Input: part model. Units: mm. Frame: model coordinates. Face numbers are marked on the shaded views. A direction names the side the tool comes from. Coordinates: 2 decimals unless noted, no trailing zeros. Write each loop counter-clockwise with the first axis right and the second up, starting at its lowest first coordinate (ties: lowest second). Pieces come first, ordered by that corner, then holes. Notation, with made-up numbers: (-38, 69) - (5, 69) arc R23 cw to (5, 102) - close; hole circle Ø9 at (-4, -32). An arc over 180 degrees is marked (long way). Put each result on its own line as item: value. Start each with the question number.
1. Cut plane A-A, the plane x = 7.5. Return loops of the section in (y, z), and give its area (3 significant figures).
2. Line query: line 1 (Y direction, x = 7.5, z = 1.5); line 2 (Y direction, x = 5.75, z = 0.85); line 3 (X direction, y = 1.5, z = 0.95). Output: solid intervals per line, ascending.
3. Access query for the marked faces 4, 5 and 6. Directions: +Z, -Z, +X, -X, +Y, -Y. A direction counts if a zero-diameter tool reaches every point of the face in a straight line with its end or side. Return the directions, or none.
4. Pin query (flat end, axial travel): pin 1 (0.9 mm diameter, centred on x = 4.5, z = 1, fed in from -Y); pin 2 (0.7 mm diameter, centred on y = -0.5, z = 2, fed in from +X). Return the tip coordinate at first contact, or that it passes through.
5. Pull-direction query (Z, two-part tool) for the marked faces 1, 2 and 3; classes: released by +Z, released by -Z, zero draft, split by the parting line, or undercut.
6. Cut plane B-B, the plane x = 1. Return loops of the section in (y, z).
7. Cut plane C-C, the plane y = 1.5. Return loops of the section in (x, z), and give its area (3 significant figures).
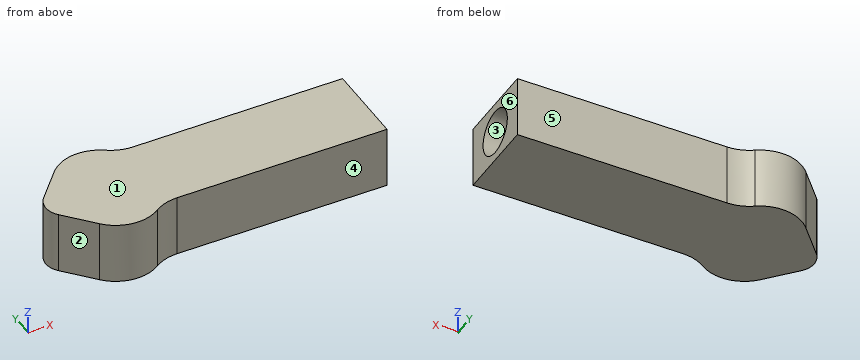
from build123d import *

# Parameters (mm, degrees)
BOSS_EXTRUDE1_DEPTH     = 3
FILLET2_R               = 2
FILLET3_R               = 2
M1_6_TAPPED_HOLE1_D     = 1.25
M1_6_TAPPED_HOLE1_DEPTH = 3
M1_6_TAPPED_HOLE1_TIP   = 0.375537887
SKETCH5_R               = 1.0922
CUT_EXTRUDE1_DEPTH      = 3


with BuildPart() as part:
    # Sketch1 → Boss-Extrude1 (new body)
    with BuildSketch(Plane.XY):
        with BuildLine():
            Line((-3.05, 2), (-3.05, 4))
            Line((-3.05, 4), (-6.05, 0.669251394))
            ThreePointArc((-6.05, 0.669251394), (-6.30696395, 0), (-6.05, -0.669251394))
            Line((-6.05, -0.669251394), (-3.05, -4))
            Line((-3.05, -4), (-3.05, -2))
            Line((-3.05, -2), (3.05, -2))
            Line((3.05, -2), (9.05, -2))
            Line((9.05, -2), (9.05, 2))
            Line((9.05, 2), (3.05, 2))
            Line((3.05, 2), (-3.05, 2))
        make_face()
    extrude(amount=BOSS_EXTRUDE1_DEPTH)

    # Fillet2
    fillet2_edges = [part.edges().sort_by_distance(p)[0] for p in [
        (-3.05, -2, 1.5),
        (-3.05, 2, 1.5),
    ]]
    fillet(fillet2_edges, radius=FILLET2_R - 0.0001)  # a hair under: the kernel refuses the full size

    # Fillet3
    fillet3_edges = [part.edges().sort_by_distance(p)[0] for p in [
        (-3.05, 4, 1.5),
        (-3.05, -4, 1.5),
    ]]
    fillet(fillet3_edges, radius=FILLET3_R)

    # M1.6 Tapped Hole1
    with Locations(Plane(origin=(9.05, 0, 0), x_dir=(0, 0, -1), z_dir=(1, 0, 0))):
        with Locations((-1.5, 0)):
            Hole(M1_6_TAPPED_HOLE1_D / 2, depth=M1_6_TAPPED_HOLE1_DEPTH)
            with Locations((0, 0, -(M1_6_TAPPED_HOLE1_DEPTH + M1_6_TAPPED_HOLE1_TIP / 2))):  # 118° drill point
                Cone(0, M1_6_TAPPED_HOLE1_D / 2, M1_6_TAPPED_HOLE1_TIP, mode=Mode.SUBTRACT)

    # Sketch5 → Cut-Extrude1 (cut)
    with BuildSketch(Plane(origin=(9.05, 0, 0), x_dir=(0, 0, -1), z_dir=(1, 0, 0))):
        with Locations((-1.5, 0)):
            Circle(SKETCH5_R)
    extrude(amount=-CUT_EXTRUDE1_DEPTH, mode=Mode.SUBTRACT)


solid = part.part
Report:
1. outline: (-2, 0) - (2, 0) - (2, 3) - (-2, 3) - close; hole circle Ø2.18 at (0, 1.5)
1. area: 8.25 mm^2
2. line 1: y = -2 to -1.09, 1.09 to 2
2. line 2: y = -2 to 2
2. line 3: x = -5.3 to 9.05
3. face 4: +Z, -Z, +X, -Y
3. face 5: +Z, -Z, +X, +Y
3. face 6: +Z, -Z, +X, +Y, -Y
4. pin 1: stops at y = -2
4. pin 2: stops at x = 6.05
5. face 1: released by +Z
5. face 2: zero draft
5. face 3: undercut
6. outline: (-2, 0) - (2, 0) - (2, 3) - (-2, 3) - close
7. outline: (-5.3, 0) - (9.05, 0) - (9.05, 3) - (-5.3, 3) - close
7. area: 43.1 mm^2
